Work out the finished part from the listing and answer in its coordinate system (mm). Face numbers are marked on the shaded views. Round coordinates to 2 decimals unless told otherwise and drop trailing zeros. Write each loop counter-clockwise with the first axis right and the second up, starting at its lowest first coordinate (ties: lowest second). Pieces come first, ordered by that corner, then holes. Notation, with made-up numbers: (55, 25.25) -> (81, 25.25) arc R11 cw to (81, 41.25) -> close; hole circle Ø11 at (4.25, -8). An arc over 180 degrees is marked (long way). One line per item, written item: value.
```python
from build123d import *

# Parameters (mm, degrees)
SKETCH1_W     = 5
SKETCH1_H     = 19
CHAMFER1_SIZE = 2.5
CHAMFER2_SIZE = 2.5


with BuildPart() as part:
    # Sketch1 → Revolve1 (revolve)
    with BuildSketch(Plane.XY, mode=Mode.PRIVATE) as revolve1_sk:
        with Locations((-7.5, 2.799270073)):
            Rectangle(SKETCH1_W, SKETCH1_H)
    revolve(revolve1_sk.sketch.rotate(Axis((0, 14.390243325, 0), (0, -1, 0)), 270), axis=Axis((0, 14.390243325, 0), (0, -1, 0)))

    # Chamfer1
    chamfer1_edges = [part.edges().sort_by_distance(p)[0] for p in [
        (0, 12.299270073, -10),
    ]]
    chamfer(chamfer1_edges, length=CHAMFER1_SIZE)

    # Chamfer2
    chamfer2_edges = [part.edges().sort_by_distance(p)[0] for p in [
        (0, -6.700729927, -10),
    ]]
    chamfer(chamfer2_edges, length=CHAMFER2_SIZE)


solid = part.part
```
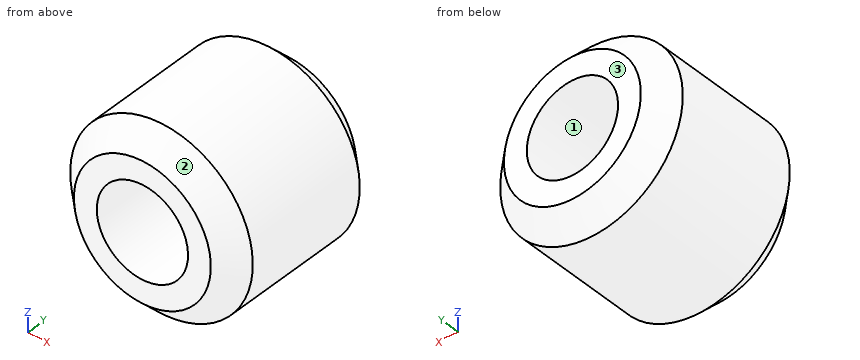
(1) Find section D-D on y = 10.5. Give the vertices of the cut face in (x, z).
Reported:
outline: circle Ø18.6 at (0, 0); hole circle Ø10 at (0, 0)
(2) Consider probe 1 along X at (y, z) = (6.5, 0); probe 2 along Z at (x, y) = (-4.25, 1.5); probe 3 along X at (y, z) = (3, -4). Determine where each line is inside the solid, lowest interval first.
Reported:
probe 1: x = -10 to -5, 5 to 10
probe 2: z = -9.05 to -2.63, 2.63 to 9.05
probe 3: x = -9.17 to -3, 3 to 9.17
(3) Find section C-C on y = 6.75. Give the vertices of the cut face in (x, z), plus the area to 3 significant figures.
Reported:
outline: circle Ø20 at (0, 0); hole circle Ø10 at (0, 0)
area: 236 mm2
(4) Find section B-B on z = 0. Give the vertices of the cut face in (x, y).
Reported:
outline: (-10, -4.2) -> (-7.5, -6.7) -> (-5, -6.7) -> (-5, 12.3) -> (-7.5, 12.3) -> (-10, 9.8) -> close; (5, -6.7) -> (7.5, -6.7) -> (10, -4.2) -> (10, 9.8) -> (7.5, 12.3) -> (5, 12.3) -> close
(5) Flat-ended cylindrical pins translate along their axes: pin 1 Ø5 at (y, z) = (-4, -3.5) entering from +X; pin 2 Ø1.5 at (x, y) = (6.5, -4.5) entering from -Z; pin 3 Ø3 at (x, y) = (4.5, 7.5) entering from -Z. Find the tip coordinate at first contact, or state that the pin passes through.
Reported:
pin 1: stops at x = 9.95
pin 2: stops at z = -8.14
pin 3: stops at z = -9.54
(6) Find section A-A on x = 0. Give the vertices of the cut face in (y, z), plus the area to 4 significant figures.
Reported:
outline: (-6.7, -7.5) -> (-4.2, -10) -> (9.8, -10) -> (12.3, -7.5) -> (12.3, -5) -> (-6.7, -5) -> close; (-6.7, 5) -> (12.3, 5) -> (12.3, 7.5) -> (9.8, 10) -> (-4.2, 10) -> (-6.7, 7.5) -> close
area: 177.5 mm2
(7) For a pull along Z with two mould halves and no side action, classify the marked faces 1, 2 and 3 as pulls with the +Z half, pulls with the -Z half, needs draft (parallel to the pull), parting line crosses it, or undercut.
Reported:
face 1: undercut
face 2: parting line crosses it
face 3: needs draft
